Study the drawing (mm; zero at the part's minimum x, y, z) and answer. A direction names the side the tool comes from. Coordinates: 2 decimals unless noted, no trailing zeros. Order: outer loops, then holes, each group sorted by start corner. A loop starts at its lowest first (then second) coordinate and runs counter-clockwise, first axis right, second up.
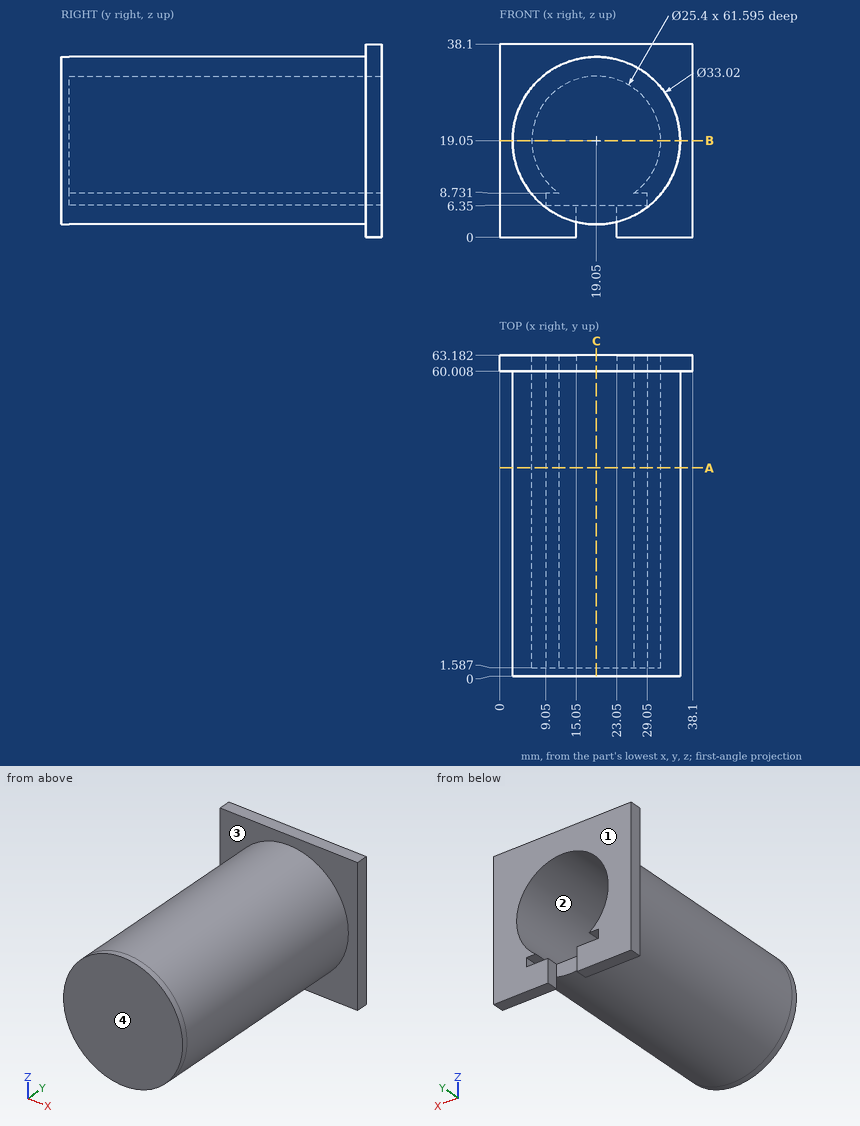
1) Flat-ended cylindrical pins translate along their axes: pin 1 Ø0.8 at (x, y) = (9.5, 25) entering from -Z; pin 2 Ø1.5 at (x, y) = (16, 18) entering from -Z; pin 3 Ø2.5 at (y, z) = (45.5, 7) entering from +X. Find the tip coordinate at first contact, or state that the pin passes through.
A:
pin 1: stops at z = 5.31
pin 2: stops at z = 2.7
pin 3: stops at x = 31.54
2) A cutting plane is placed at B-B, the plane z = 19.05. Determine the outline of the cut face in (x, y).
A:
outline: (0, 60.01) - (2.54, 60.01) - (2.54, 0) - (35.56, 0) - (35.56, 60.01) - (38.1, 60.01) - (38.1, 63.18) - (31.75, 63.18) - (31.75, 1.59) - (6.35, 1.59) - (6.35, 63.18) - (0, 63.18) - close
3) Straight lines are drawn through the part: line 1 (Z direction, x = 19.05, y = 20); line 2 (Y direction, x = 16, z = 19). For each, find the intervals that lie inside material, in ascending order.
A:
line 1: z = 2.54 to 6.35, 31.75 to 35.56
line 2: y = 0 to 1.59
4) Determine the mould class of the marked faces 1 and 2 for opening direction X: pulls with the +X half, pulls with the -X half, needs draft (parallel to the pull), parting line crosses it, or undercut.
A:
face 1: needs draft
face 2: undercut
5) A cutting plane is placed at A-A, the plane y = 41. Determine the outline of the cut face in (x, z), and give its area (3 significant figures).
A:
outline: circle Ø33.02 at (19.05, 19.05); hole (9.05, 6.35) - (29.05, 6.35) - (29.05, 8.73) - (26.45, 8.73) arc R12.7 ccw (long way) to (11.65, 8.73) - (9.05, 8.73) - close
area: 326 mm2
6) A cutting plane is placed at C-C, the plane x = 19.05. Determine the outline of the cut face in (y, z).
A:
outline: (0, 2.54) - (60.01, 2.54) - (60.01, 6.35) - (1.59, 6.35) - (1.59, 31.75) - (63.18, 31.75) - (63.18, 38.1) - (60.01, 38.1) - (60.01, 35.56) - (0, 35.56) - close
7) Which of the six approach directions +Z, -Z, +X, -X, +Y, -Y give full straight-line access (tool end or side, diameter ignored) to the marked faces 3 and 4?
A:
face 3: -Y
face 4: +Z, -Z, +X, -X, -Y
